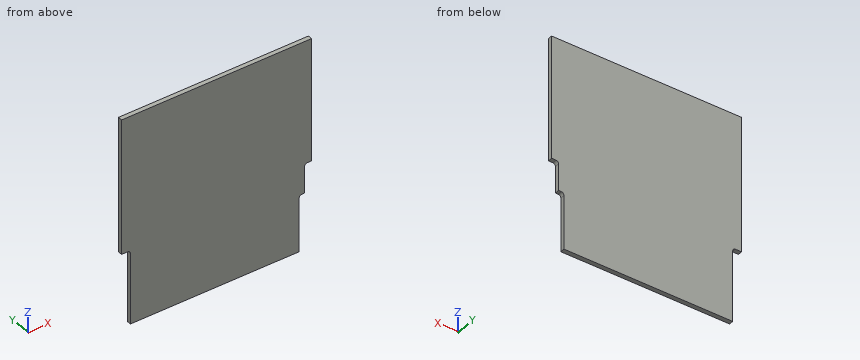
from build123d import *

# Parameters (mm, degrees)
FR4_DEPTH = 1.5875


with BuildPart() as part:
    # Sketch1 → FR4 (new body)
    with BuildSketch(Plane(origin=(0, 0, 0), x_dir=(1, 0, 0), z_dir=(0, 1, 0))):
        with BuildLine():
            Line((-34.5, -9), (34.5, -9))
            Line((34.5, -9), (34.5, 36))
            Line((34.5, 36), (32.940007652, 36))
            ThreePointArc((32.940007652, 36), (32.271894631, 36.313775841), (32, 37))
            Line((32, 37), (32, 46.75))
            Line((32, 46.75), (31, 46.75))
            ThreePointArc((31, 46.75), (30.292893219, 47.042893219), (30, 47.75))
            Line((30, 47.75), (30, 67.5))
            Line((30, 67.5), (-31.3, 67.5))
            Line((-31.3, 67.5), (-31.3, 41.5))
            ThreePointArc((-31.3, 41.5), (-31.564481186, 40.821086647), (-32.218527823, 40.5))
            Line((-32.218527823, 40.5), (-34.5, 40.5))
            Line((-34.5, 40.5), (-34.5, -9))
        make_face()
    extrude(amount=FR4_DEPTH)


solid = part.part
Geometry: final body of the model. Coordinates: model frame, mm. Round coordinates to 2 decimals unless told otherwise and drop trailing zeros. Loops run counter-clockwise (first coordinate to the right, second up) from the corner with the lowest first, then second, coordinate; pieces in that order, holes last.
Q1. Material intervals for L1, parallel to X at y = 0.2, z = -63; L2, parallel to X at y = 0.7, z = -38, sorted ascending.
Q2. Section A-A on y = 0.5. Return loops of the section in (x, z).
Q3. Section B-B on z = -58. Return loops of the section in (x, y).
Q4. Pin query (flat end, axial travel): P1, Ø0.8, axis at y = 1, z = -58.5, coming from the +X side; P2, Ø0.8, axis at x = 31.5, y = 1, coming from the -Z side; P3, Ø0.5, axis at x = -33.5, y = 0.5, coming from the -Z side. Return the tip coordinate at first contact, or that it passes through.
Q5. Section C-C on z = -44.5. Return loops of the section in (x, y).
Evaluation:
1. L1: x = -31.3 to 30
1. L2: x = -34.5 to 32
2. outline: (-34.5, -40.5) - (-32.22, -40.5) arc R1 cw to (-31.3, -41.5) - (-31.3, -67.5) - (30, -67.5) - (30, -47.75) arc R1 cw to (31, -46.75) - (32, -46.75) - (32, -37) arc R1 cw to (32.94, -36) - (34.5, -36) - (34.5, 9) - (-34.5, 9) - close
3. outline: (-31.3, 0) - (30, 0) - (30, 1.59) - (-31.3, 1.59) - close
4. P1: stops at x = 30
4. P2: stops at z = -46.75
4. P3: stops at z = -40.5
5. outline: (-31.3, 0) - (32, 0) - (32, 1.59) - (-31.3, 1.59) - close
